```python
from build123d import *

# Parameters (mm, degrees)
SKETCH1_R           = 1.5
SKETCH1_R_2         = 2.25
BOSS_EXTRUDE1_DEPTH = 3


with BuildPart() as part:
    # Sketch1 → Boss-Extrude1 (new body)
    with BuildSketch(Plane.XY):
        with BuildLine():
            Line((-13.25, 27.95), (13.25, 27.95))
            ThreePointArc((13.25, 27.95), (15.371320344, 27.071320344), (16.25, 24.95))
            Line((16.25, 24.95), (16.25, -24.95))
            ThreePointArc((16.25, -24.95), (15.371320344, -27.071320344), (13.25, -27.95))
            Line((13.25, -27.95), (-13.25, -27.95))
            ThreePointArc((-13.25, -27.95), (-15.371320344, -27.071320344), (-16.25, -24.95))
            Line((-16.25, -24.95), (-16.25, 24.95))
            ThreePointArc((-16.25, 24.95), (-15.371320344, 27.071320344), (-13.25, 27.95))
        make_face()
        with Locations((5, 24.45)):
            Circle(SKETCH1_R, mode=Mode.SUBTRACT)
        with Locations(Location((5, -24.45, 0), (0, 0, 180))):
            Circle(SKETCH1_R, mode=Mode.SUBTRACT)
        with Locations(Location((-5, -24.45, 0), (0, 0, 180))):
            Circle(SKETCH1_R_2, mode=Mode.SUBTRACT)
        with BuildLine():
            Line((-10.25, 20.45), (-3.5, 20.45))
            Line((-3.5, 20.45), (-3.5, 22.772949017))
            ThreePointArc((-3.5, 22.772949017), (-7.053959591, 25.368558654), (-2.75, 24.45))
            Line((-2.75, 24.45), (2.5, 24.45))
            ThreePointArc((2.5, 24.45), (3.207106781, 24.157106781), (3.5, 23.45))
            Line((3.5, 23.45), (3.5, 20.45))
            Line((3.5, 20.45), (10.25, 20.45))
            Line((10.25, 20.45), (10.25, 15.45))
            Line((10.25, 15.45), (13.25, 15.45))
            Line((13.25, 15.45), (13.25, 10.45))
            Line((13.25, 10.45), (10.25, 10.45))
            Line((10.25, 10.45), (10.25, 5.45))
            Line((10.25, 5.45), (13.25, 5.45))
            Line((13.25, 5.45), (13.25, 0.45))
            Line((13.25, 0.45), (10.25, 0.45))
            Line((10.25, 0.45), (10.25, -20.45))
            Line((10.25, -20.45), (-10.25, -20.45))
            Line((-10.25, -20.45), (-10.25, 0.45))
            Line((-10.25, 0.45), (-13.25, 0.45))
            Line((-13.25, 0.45), (-13.25, 5.45))
            Line((-13.25, 5.45), (-10.25, 5.45))
            Line((-10.25, 5.45), (-10.25, 10.45))
            Line((-10.25, 10.45), (-13.25, 10.45))
            Line((-13.25, 10.45), (-13.25, 15.45))
            Line((-13.25, 15.45), (-10.25, 15.45))
            Line((-10.25, 15.45), (-10.25, 20.45))
        make_face(mode=Mode.SUBTRACT)
    extrude(amount=BOSS_EXTRUDE1_DEPTH)


solid = part.part
```
Geometry check sheet. Reference: the model listing, model coordinates, mm. A direction names the side the tool comes from. Coordinates: 2 decimals unless noted, no trailing zeros. Write each loop counter-clockwise with the first axis right and the second up, starting at its lowest first coordinate (ties: lowest second). Pieces come first, ordered by that corner, then holes. Notation, with made-up numbers: M 43.25,-17 L 73.25,-17 A19 cw 73.25,7 Z; hole C 72,46.25 d7. An arc over 180 degrees is marked long. Answer as a JSON object with one key per item and string values.
1. Scan lines: L1, parallel to Y at x = 5, z = 0.6; L2, parallel to Y at x = -5, z = 0.9; L3, parallel to X at y = -24.45, z = 1.95. Record each from-to range of solid material in increasing order.
Answers below:
{"L1": "y = -27.95 to -25.95, -22.95 to -20.45, 20.45 to 22.95, 25.95 to 27.95", "L2": "y = -27.95 to -26.7, -22.2 to -20.45, 20.45 to 22.2, 26.7 to 27.95", "L3": "x = -16.25 to -7.25, -2.75 to 3.5, 6.5 to 16.25"}
2. Section check D-D, the plane z = 2.2. Give the number of separate pieces and of enclosed holes in the cut face, plus the area to 3 significant figures.
Answers below:
{"separate pieces": "1", "enclosed holes": "4", "area": "838 mm²"}
3. Section check B-B, the plane y = 18.5. Enter the section's corners in (x, z).
Answers below:
{"outline": "M -16.25,0 L -10.25,0 L -10.25,3 L -16.25,3 Z; M 10.25,0 L 16.25,0 L 16.25,3 L 10.25,3 Z"}
4. Tool access check on faces 1 (the flat face through (12, 15.45, 1)), 2 (the flat face through (-16.25, 0, 1)). Record the directions out of +Z, -Z, +X, -X, +Y, -Y that give a thin tool (end or side, any length) a straight path to the whole face; none if there is none.
Answers below:
{"face 1": "+Z, -Z", "face 2": "+Z, -Z, -X, +Y, -Y"}
5. Section check A-A, the plane x = -8.5. Enter the section's corners in (y, z), plus the area to 3 significant figures.
Answers below:
{"outline": "M -27.95,0 L -20.45,0 L -20.45,3 L -27.95,3 Z; M 20.45,0 L 27.95,0 L 27.95,3 L 20.45,3 Z", "area": "45.0 mm²"}
6. Section check C-C, the plane x = 5. Enter the section's corners in (y, z), plus the area to 3 significant figures.
Answers below:
{"outline": "M -27.95,0 L -25.95,0 L -25.95,3 L -27.95,3 Z; M -22.95,0 L -20.45,0 L -20.45,3 L -22.95,3 Z; M 20.45,0 L 22.95,0 L 22.95,3 L 20.45,3 Z; M 25.95,0 L 27.95,0 L 27.95,3 L 25.95,3 Z", "area": "27.0 mm²"}
7. Draft check along Y on faces 3 (the flat face through (3.5, 22, 1)), 4 (the flat face through (16.25, 0, 1)), 5 (the cylindrical face through (-15.39, 27.05, 1.48)). Enter one of: released by +Y, released by -Y, zero draft, split by the parting line, or undercut.
Answers below:
{"face 3": "undercut", "face 4": "zero draft", "face 5": "released by +Y"}
8. Go/stop test with a flat-tipped pin: pin 1 Ø10 at (x, y) = (-2.5, -2.5) entering from -Z. Record where the tip stops, or that it passes through.
Answers below:
{"pin 1": "passes through"}
